Autodesk Inventor part; units mm, degrees
ref_plane "YZ Plane" through (0, 0, 0) normal (1, 0, 0) x (0, 1, 0)
ref_plane "XZ Plane" through (0, 0, 0) normal (0, 1, 0) x (-1, 0, 0)
ref_plane "XY Plane" through (0, 0, 0) normal (0, 0, 1) x (1, 0, 0)
sketch "Sketch1" plane through (0, 0, 0) normal (0, 0, 1) x (1, 0, 0)
  line L0 (0, 0) -> (43, 0)
  line L1 (43, 0) -> (43, 20)
  line L2 (43, 20) -> (0, 20)
  line L3 (0, 20) -> (0, 0)
  circle A0 centre (10, 10) radius 1.6
  circle A1 centre (33, 10) radius 1.6
  line L4 (0, -10) -> (10, -10)
  line L5 (10, -10) -> (10, 0)
  line L6 (10, 0) -> (0, 0)
  line L7 (0, 0) -> (0, -10)
  circle A2 centre (5, -5) radius 1.5
  point P0 (0, 10)
  point P1 (0, -5)
  point P2 (5, 0)
  dimension "d2" = 20
  dimension "d3" = 3.2
  dimension "d4" = 3.2
  dimension "d5" = 10
  dimension "d6" = 10
  dimension "d10" = 23
  dimension "d15" = 10
  dimension "d16" = 10
  dimension "d17" = 3
extrude "Extrusion1" add sketch "Sketch1" along normal blind 5
sketch "Sketch2" plane through (0, 0, 5) normal (0, 0, 1) x (1, 0, 0)
  circle A0 centre (10, 10) radius 1.6
  circle A1 centre (10, 10) radius 5
  point P0 (0, 0)
  dimension "d11" = 10
extrude "Extrusion2" add sketch "Sketch2" along normal blind 1.6
fillet "Fillet2" radius 5 6 edges at (43, 20, 2.5) (43, 0, 2.5) (10, -10, 2.5) (0, -10, 2.5) (10, 0, 2.5) (0, 20, 2.5)
sketch "Sketch3" plane through (0, 0, 5) normal (0, 0, 1) x (1, 0, 0)
  line L0 (0, 0) -> (16.7828, 0)
  line L1 (16.7828, 0) -> (16.7828, -11.2372)
  line L2 (16.7828, -11.2372) -> (0, -11.2372)
  line L3 (0, -11.2372) -> (0, 0)
extrude "Extrusion3" cut sketch "Sketch3" against normal blind 2.5
fillet "Fillet3" radius 5 1 edges at (0, 0, 3.75)
properties part number "wheel tensioner"
Work out the finished part from the listing and answer in its coordinate system (mm). A direction names the side the tool comes from. Give positions to 0.01 mm unless a question says otherwise; leave off trailing zeros. Loops run counter-clockwise (first coordinate to the right, second up) from the corner with the lowest first, then second, coordinate; pieces in that order, holes last. Notation, with made-up numbers: (-36.5, 60.25) - (17.5, 60.25) arc R13 ccw to (17.5, 74.25) - close; hole circle Ø3 at (43, 67.25). An arc over 180 degrees is marked (long way). Answer in a Markdown table with one row per item.
(1) Section B-B (z = 1) is taken. State how many separate pieces and enclosed holes the cut face has, and give its area (3 significant figures).
Results list:
| item | result |
|---|---|
| separate pieces | 1 |
| enclosed holes | 3 |
| area | 915 mm² |
(2) A tool of negligible diameter and unlimited length cuts with its end or side. For faces 1 (the face through (2, 1, 4)), 2 (the face through (25, 0, 2)), 3 (the face through (14.77, 8.5, 5.79)), 4 (the face through (12, -1, 1)), from which of +Z, -Z, +X, -X, +Y, -Y can it reach the whole face along a straight path? Write none if from no direction.
Results list:
| item | result |
|---|---|
| face 1 | +Z, -X, -Y |
| face 2 | +Z, +X, -Y |
| face 3 | +Z |
| face 4 | +Z, -Z, +X, -Y |
(3) For a pull along X with two mould halves and no side action, classify faces 5 (the face through (43, 10, 2)), 6 (the face through (8.73, 10.97, 3.25)), 7 (the face through (22, 20, 2)) as pulls with the +X half, pulls with the -X half, needs draft (parallel to the pull), parting line crosses it, or undercut.
Results list:
| item | result |
|---|---|
| face 5 | pulls with the +X half |
| face 6 | undercut |
| face 7 | needs draft |
(4) Consider L1, parallel to Y at x = 5, z = 0.9; L2, parallel to X at y = 10.75, z = 3; L3, parallel to Z at x = 36.5, y = 4.5. Determine where each line is inside the solid, lowest interval first. Write a range as [from, to].
Results list:
| item | result |
|---|---|
| L1 | y = [-10, -6.5], [-3.5, 20] |
| L2 | x = [0, 8.59], [11.41, 31.59], [34.41, 43] |
| L3 | z = [0, 5] |
(5) Section D-D (y = 6) is taken. Give the vertices of the cut face in (x, z), and give its area (3 significant figures).
Results list:
| item | result |
|---|---|
| outline | (0, 0) - (43, 0) - (43, 5) - (13, 5) - (13, 6.6) - (7, 6.6) - (7, 5) - (0, 5) - close |
| area | 225 mm² |
(6) Section A-A (y = 10) is taken. Give the vertices of the cut face in (x, z), and give its area (3 significant figures).
Results list:
| item | result |
|---|---|
| outline | (0, 0) - (8.4, 0) - (8.4, 6.6) - (5, 6.6) - (5, 5) - (0, 5) - close; (11.6, 0) - (31.4, 0) - (31.4, 5) - (15, 5) - (15, 6.6) - (11.6, 6.6) - close; (34.6, 0) - (43, 0) - (43, 5) - (34.6, 5) - close |
| area | 194 mm² |
(7) Flat-ended cylindrical pins translate along their axes: pin 1 Ø12 at (x, y) = (35.5, 0.5) entering from +Z; pin 2 Ø4 at (x, y) = (10, 10) entering from -Z; pin 3 Ø2 at (x, z) = (20, 1.5) entering from -Y; pin 4 Ø1.5 at (y, z) = (17, 1) entering from -X. Find the tip coordinate at first contact, or state that the pin passes through.
Results list:
| item | result |
|---|---|
| pin 1 | stops at z = 5 |
| pin 2 | stops at z = 0 |
| pin 3 | stops at y = 0 |
| pin 4 | stops at x = 0.16 |
(8) Section C-C (x = 33) is taken. Give the vertices of the cut face in (y, z).
Results list:
| item | result |
|---|---|
| outline | (0, 0) - (8.4, 0) - (8.4, 5) - (0, 5) - close; (11.6, 0) - (20, 0) - (20, 5) - (11.6, 5) - close |
